from build123d import *

# Parameters (mm, degrees)
F1_DEPTH = 47.244
F2_DEPTH = 4.826
F4_DEPTH = 5.08


with BuildPart() as f1:
    # F0 (on Top) → F1 (new body)
    with BuildSketch(Plane.XY):
        with BuildLine():
            Line((-22.916476, 21.291338), (-22.916476, 29.532059))
            ThreePointArc((-22.916476, 29.532059), (-37.380167, 0.174641), (-23.191419, -29.316641))
            Line((-23.191419, -29.316641), (-22.916476, -29.316641))
            Line((-22.916476, -29.316641), (-22.916476, -21.291338))
            ThreePointArc((-22.916476, -21.291338), (-31.28076, 0), (-22.916476, 21.291338))
        make_face()
        with BuildLine():
            ThreePointArc((-23.191419, -29.316641), (16.284944, -33.646812), (37.380575, 0))
            ThreePointArc((37.380575, 0), (16.441963, 33.570362), (-22.916476, 29.532059))
            Line((-22.916476, 29.532059), (-22.916476, 21.291338))
            ThreePointArc((-22.916476, 21.291338), (11.437683, 29.114693), (31.28076, 0))
            ThreePointArc((31.28076, 0), (11.437683, -29.114693), (-22.916476, -21.291338))
            Line((-22.916476, -21.291338), (-22.916476, -29.316641))
            Line((-22.916476, -29.316641), (-23.191419, -29.316641))
        make_face()
    extrude(amount=F1_DEPTH)

    # F0 (on Top) → F2 (join)
    with BuildSketch(Plane.XY):
        with BuildLine():
            ThreePointArc((-23.191419, -29.316641), (-37.380167, 0.174641), (-22.916476, 29.532059))
            Line((-22.916476, 29.532059), (-78.842215, 29.532059))
            Line((-78.842215, 29.532059), (-78.842215, -29.316641))
            Line((-78.842215, -29.316641), (-23.191419, -29.316641))
        make_face()
    extrude(amount=F2_DEPTH)

    # F3 (on Front) → F4 (join, symmetric)
    with BuildSketch(Plane.XZ):
        Polygon((-37.321575, 4.987057), (-37.321575, 47.026183), (-58.294769, 4.987057), align=None)
    extrude(amount=F4_DEPTH, both=True)


solid = f1.part
Design review of the part built by this model. Coordinates are the model's own, in mm. A direction names the side the tool comes from. Coordinates: 2 decimals unless noted, no trailing zeros. Loops run counter-clockwise (first coordinate to the right, second up) from the corner with the lowest first, then second, coordinate; pieces in that order, holes last. Notation, with made-up numbers: (29.5, 71.25) -> (81.5, 71.25) arc R11 ccw to (81.5, 90.25) -> close; hole circle Ø3 at (86.5, 80). An arc over 180 degrees is marked (long way). Use a Markdown table: item, result. Add a question column.
Item 1: The part is to be moulded in two halves that separate along X. For faces 6 (the flat face through (-34, 1, 0)), 7 (the flat face through (-47.66, -0.07, 26.3)), 8 (the flat face through (-37.322, 4, 26)), say which applies: +X half, -X half, draft (parallel to the pull), parting line (faces both ways), or undercut.
Item 2: Clearance check with flat-ended pins moving along their axes: P1, Ø5.5, axis at x = -46.5, z = 2.5, coming from the -Y side; P2, Ø10.5, axis at x = -46, z = 18.5, coming from the -Y side; P3, Ø5.5, axis at x = -59.5, z = 3, coming from the +Y side; P4, Ø1, axis at x = -29.5, y = 7, coming from the -Z side. State where each tip first meets the part, or that it passes through.
Item 3: We need section B-B, the plane z = 30. Write out the cut boundary in (x, y).
Item 4: Machinability: for faces 1 (the flat face through (-48, 0, 4.987)), 2 (the flat face through (-51, -29.317, 2)), 3 (the flat face through (-43, -5.08, 17)), 4 (the flat face through (-50, 29.532, 2)), 5 (the flat face through (-43, 5.08, 17)), which of the approach directions +Z, -Z, +X, -X, +Y, -Y give a long, thin tool a straight path to every point of the face, cutting with its end or side? Answer none if there is none.
Item 5: We need section C-C, the plane x = -2. Write out the cut boundary in (y, z), and give its area (3 significant figures).
Item 6: We need section D-D, the plane y = 16. Write out the cut boundary in (x, z).
Item 7: We need section A-A, the plane y = 27. Write out the cut boundary in (x, z).
Item 8: Wall thickness on L1, parallel to Z at x = -50.5, y = 13; L2, parallel to Y at x = 20.5, z = 16.5; L3, parallel to X at y = 7, z = 32: over which ranges is each line inside the solid? List them lowest first. Write a range as from..to.
Numbers:
| question | item | result |
|---|---|---|
| 1 | face 6 | draft |
| 1 | face 7 | -X half |
| 1 | face 8 | undercut |
| 2 | P1 | stops at y = -29.32 |
| 2 | P2 | stops at y = -5.08 |
| 2 | P3 | stops at y = 29.53 |
| 2 | P4 | passes through |
| 3 | outline | (-45.82, -5.08) -> (-37.32, -5.08) -> (-37.32, -2.1) arc R37.38 ccw (long way) to (-37.32, 2.1) -> (-37.32, 5.08) -> (-45.82, 5.08) -> close; hole circle Ø62.56 at (0, 0) |
| 4 | face 1 | -X, +Y, -Y |
| 4 | face 2 | +Z, -Z, -X, -Y |
| 4 | face 3 | +Z, -X, -Y |
| 4 | face 4 | +Z, -Z, -X, +Y |
| 4 | face 5 | +Z, -X, +Y |
| 5 | outline | (-37.33, 0) -> (-31.22, 0) -> (-31.22, 47.24) -> (-37.33, 47.24) -> close; (31.22, 0) -> (37.33, 0) -> (37.33, 47.24) -> (31.22, 47.24) -> close |
| 5 | area | 577 mm^2 |
| 6 | outline | (-78.84, 0) -> (-26.88, 0) -> (-26.88, 47.24) -> (-33.78, 47.24) -> (-33.78, 4.83) -> (-78.84, 4.83) -> close; (26.88, 0) -> (33.78, 0) -> (33.78, 47.24) -> (26.88, 47.24) -> close |
| 7 | outline | (-78.84, 0) -> (-15.8, 0) -> (-15.8, 47.24) -> (-25.85, 47.24) -> (-25.85, 4.83) -> (-78.84, 4.83) -> close; (15.8, 0) -> (25.85, 0) -> (25.85, 47.24) -> (15.8, 47.24) -> close |
| 8 | L1 | z = 0..4.83 |
| 8 | L2 | y = -31.26..-23.63, 23.63..31.26 |
| 8 | L3 | x = -36.72..-30.49, 30.49..36.72 |
